Design review of the part built by this model. Coordinates are the model's own, in mm. Give positions to 0.01 mm unless a question says otherwise; leave off trailing zeros. Loops run counter-clockwise (first coordinate to the right, second up) from the corner with the lowest first, then second, coordinate; pieces in that order, holes last. Notation, with made-up numbers: (-23.75, 15.25) -> (20.25, 15.25) arc R28 ccw to (20.25, 37.25) -> close; hole circle Ø10 at (35, 70.25). An arc over 180 degrees is marked (long way). Use CSV: the item, a comma, the result in double quotes. Start each with the question number.
Item 1: The part is to be moulded in two halves that separate along X. For faces 1 (the face through (21.199, 6.676, 313.055)), 2 (the face through (-5.137, -23.135, 313.055)), say which applies: +X half, -X half, draft (parallel to the pull), parting line (faces both ways), or undercut.
Item 2: Clearance check with flat-ended pins moving along their axes: pin 1 (2.5 mm diameter, centred on x = 19.5, y = -12.5, fed in from -Z); pin 2 (5 mm diameter, centred on y = -3, z = 390, fed in from -X); pin 3 (5 mm diameter, centred on y = -13, z = 128, fed in from -X); pin 4 (3 mm diameter, centred on x = -11, z = 409, fed in from -Y). State where each tip first meets the part, or that it passes through.
Item 3: We need section B-B (x = 7). State the section outline as (y, z) points, plus the area to 3 significant figures.
Item 4: We need section A-A (y = 0). State the section outline as (x, z) points (3 decimals), plus the area to 3 significant figures.
Item 5: We need section C-C (z = 68). State the section outline as (x, y) points (3 decimals), plus the area to 3 significant figures.
Item 6: Wall thickness on line 1 along Y through (x, z) = (0, 490.5) (3 decimals); line 2 along Y through (x, z) = (14, 454.5); line 3 along X through (y, z) = (-8, 382): over which ranges is each line inside the solid? List them lowest first. Write a range as from..to.
from build123d import *

# Parameters (mm, degrees)
SKETCH1_R           = 23.6982
SKETCH1_R_2         = 22.225
BOSS_EXTRUDE1_DEPTH = 635
CUT_EXTRUDE1_START  = -77.831769
SKETCH2_W           = 2
SKETCH2_H           = 30
CUT_EXTRUDE1_DEPTH  = 1.529969
CIRPATTERN2_COUNT   = 3


with BuildPart() as part:
    # Sketch1 → Boss-Extrude1 (new body)
    with BuildSketch(Plane.XY):
        Circle(SKETCH1_R)
        Circle(SKETCH1_R_2, mode=Mode.SUBTRACT)
    extrude(amount=BOSS_EXTRUDE1_DEPTH)

    # Sketch2 → Cut-Extrude1 (cut)
    with BuildSketch(Plane(origin=(0, 100, 0), x_dir=(1, 0, 0), z_dir=(0, 1, 0)).offset(CUT_EXTRUDE1_START)):
        with Locations((0.5875, -610)):
            Rectangle(SKETCH2_W, SKETCH2_H)
    cut_extrude1 = extrude(amount=CUT_EXTRUDE1_DEPTH, mode=Mode.SUBTRACT)

    # CirPattern2: Cut-Extrude1 ×3 about axis
    cirpattern2_axis = Axis((0, 0, 0), (0, 0, 1))
    for i in range(1, CIRPATTERN2_COUNT):
        add(cut_extrude1.rotate(cirpattern2_axis, i * 360 / CIRPATTERN2_COUNT), mode=Mode.SUBTRACT)


solid = part.part
Results found:
1,face 1,"undercut"
1,face 2,"parting line"
2,pin 1,"z = 0"
2,pin 2,"x = -23.69"
2,pin 3,"x = -21.25"
2,pin 4,"y = -21.71"
3,outline,"(-22.64, 0) -> (-21.09, 0) -> (-21.09, 635) -> (-22.64, 635) -> close; (21.09, 0) -> (22.64, 0) -> (22.64, 635) -> (21.09, 635) -> close"
3,area,"1,960 mm²"
4,outline,"(-23.698, 0) -> (-22.225, 0) -> (-22.225, 635) -> (-23.698, 635) -> close; (22.225, 0) -> (23.698, 0) -> (23.698, 635) -> (22.225, 635) -> close"
4,area,"1,870 mm²"
5,outline,"circle Ø47.396 at (0, 0); hole circle Ø44.45 at (0, 0)"
5,area,"213 mm²"
6,line 1,"-23.698..-22.225, 22.225..23.698"
6,line 2,"-19.12..-17.26, 17.26..19.12"
6,line 3,"-22.31..-20.74, 20.74..22.31"
